For this review, take the finished solid that the model builds, in its own axes (mm). A direction names the side the tool comes from. Round coordinates to 2 decimals unless told otherwise and drop trailing zeros. Write each loop counter-clockwise with the first axis right and the second up, starting at its lowest first coordinate (ties: lowest second). Pieces come first, ordered by that corner, then holes. Notation, with made-up numbers: M -9.75,44.5 L 15.25,44.5 A26 ccw 15.25,64.5 Z; hole C -33,25.5 d1. An arc over 180 degrees is marked long. One line per question, with ' | ' between items.
```python
from build123d import *

# Parameters (mm, degrees)
F0_R     = 1
F0_R_2   = 5
F0_R_3   = 4
F1_DEPTH = 2


with BuildPart() as f1:
    # F0 (on Top) → F1 (new body)
    with BuildSketch(Plane.XY):
        with BuildLine():
            Line((5, 10), (-5, 10))
            ThreePointArc((-5, 10), (-8.535534, 8.535534), (-10, 5))
            Line((-10, 5), (-10, -5))
            ThreePointArc((-10, -5), (-8.535534, -8.535534), (-5, -10))
            Line((-5, -10), (5, -10))
            ThreePointArc((5, -10), (8.535534, -8.535534), (10, -5))
            Line((10, -5), (10, 5))
            ThreePointArc((10, 5), (8.535534, 8.535534), (5, 10))
        make_face()
        with Locations((-6.75, -6.75)):
            Circle(F0_R, mode=Mode.SUBTRACT)
        with Locations((6.75, -6.75)):
            Circle(F0_R, mode=Mode.SUBTRACT)
        with Locations((-6.75, 6.75)):
            Circle(F0_R, mode=Mode.SUBTRACT)
        Circle(F0_R_2, mode=Mode.SUBTRACT)
        with Locations((6.75, 6.75)):
            Circle(F0_R, mode=Mode.SUBTRACT)
        Circle(F0_R_2)
        Circle(F0_R_3, mode=Mode.SUBTRACT)
        Circle(F0_R_3)
    extrude(amount=F1_DEPTH)

    # F3: sweep along a path in F2
    with BuildLine(Plane.YZ) as f3_path:
        Line((4, 0), (8.663077, 10))
    # F0 (on Top) → F3 (sweep)
    with BuildSketch(Plane.XY):
        Circle(F0_R_2)
        Circle(F0_R_3, mode=Mode.SUBTRACT)
        Circle(F0_R_3)
    sweep(path=f3_path.line)

    # F4: sweep along a path in F2
    with BuildLine(Plane.YZ) as f4_path:
        Line((4, 0), (8.663077, 10))
    # F0 (on Top) → F4 (sweep, cut)
    with BuildSketch(Plane.XY):
        Circle(F0_R_3)
    sweep(path=f4_path.line, mode=Mode.SUBTRACT)


solid = f1.part
```
Item 1: Insertion check: pin 1 Ø6 at (x, y) = (1, -4) entering from +Z; pin 2 Ø2.5 at (x, y) = (6.75, -6.75) entering from +Z. Each pin has a flat end and moves straight along its axis. Give the tip position at first contact, or say it passes through.
Results:
pin 1: z = 8.44 | pin 2: z = 2
Item 2: Machinability: for faces 4 (the face through (6.013, 7.426, 0.986)), 5 (the face through (-0.1, -4.3, 2)), which of the approach directions +Z, -Z, +X, -X, +Y, -Y give a long, thin tool a straight path to every point of the face, cutting with its end or side? Answer none if there is none.
Results:
face 4: +Z, -Z | face 5: none
Item 3: Take a section at C-C (y = 6.75). State how many separate pieces and enclosed holes the cut face has, then the cut area to 3 significant figures.
Results:
separate pieces: 4 | enclosed holes: 0 | area: 51.7 mm2
Item 4: To check wall thickness, follow line 1 along Y through (x, z) = (-6.75, 0.85); line 2 along X through (y, z) = (1.25, 2.25); line 3 along Z through (x, y) = (8.5, 7.25). State the ranges of each line that lie inside material, in increasing order. Write a range as from..to.
Results:
line 1: -9.68..-7.75, -5.75..5.75, 7.75..9.68 | line 2: -5..-3.99, 3.99..5 | line 3: 0..2
Item 5: Take a section at A-A (y = -6.75). Write out the cut boundary in (x, z), then the cut area to 3 significant figures.
Results:
outline: M -9.68,0 L -7.75,0 L -7.75,2 L -9.68,2 Z; M -5.75,0 L 5.75,0 L 5.75,2 L -5.75,2 Z; M 7.75,0 L 9.68,0 L 9.68,2 L 7.75,2 Z | area: 30.7 mm2
Item 6: Mouldability with a two-part tool opening along Y and no side actions: class faces 1 (the face through (-7.487, -6.074, 0.986)), 2 (the face through (-8, 9, 1)), 3 (the face through (10, 0, 1)) as +Y half, -Y half, draft (parallel to the pull), parting line (faces both ways), or undercut.
Results:
face 1: undercut | face 2: +Y half | face 3: draft
Item 7: Take a section at D-D (x = 5.25). Write out the cut boundary in (y, z), then the cut area to 3 significant figures.
Results:
outline: M -9.99,0 L 9.99,0 L 9.99,2 L -9.99,2 Z | area: 40.0 mm2
